Can you work these out from the model? Positions are in its coordinate system, mm. A direction names the side the tool comes from. Coordinates: 2 decimals unless noted, no trailing zeros. Loops run counter-clockwise (first coordinate to the right, second up) from the corner with the lowest first, then second, coordinate; pieces in that order, holes last.
Autodesk Fusion 360 part; units mm, degrees
box "BoxPrimitive1" add length 40 width 165 height 3.5 placed x (0, 1, 0) y (-1, 0, 0) z (0, 0, 1) at (165, 0, 0)
box "BoxPrimitive2" add length 40 width 2.5 height 23 placed x (0, 1, 0) y (-1, 0, 0) z (0, 0, 1) at (167.5, 0, 0)
hole "Hole1" at (167.5, 20.3218, 13.4545) direction (-1, 0, 0) diameter 6 depth 5 tip angle 180
Item 1: We'd pull the mould along Z, two halves only. Please class faces 1 (the face through (166.232, 17.792, 11.842)), 2 (the face through (84, 40, 1)), 3 (the face through (83, 20, 0)): +Z half, -Z half, draft (parallel to the pull), parting line (faces both ways), or undercut.
Results are:
face 1: undercut
face 2: draft
face 3: -Z half
Item 2: Suppose I cut it at B-B, the plane x = 42. Please give me the cut outline in (y, z).
Results are:
outline: (0, 0) - (40, 0) - (40, 3.5) - (0, 3.5) - close
Item 3: I need wall thicknesses on line 1 along Z through (x, y) = (43, 28); line 2 along X through (y, z) = (22, 17). Which ranges of each line are inside material? Lowest first, please.
Results are:
line 1: z = 0 to 3.5
line 2: x = 165 to 167.5
Item 4: Suppose I cut it at C-C, the plane z = 21.5. Please give me the cut outline in (x, y), plus the area to 3 significant figures.
Results are:
outline: (165, 0) - (167.5, 0) - (167.5, 40) - (165, 40) - close
area: 100 mm2
Item 5: On a 3-axis mill with a long thin cutter (end or side, diameter ignored), from which of +Z, -Z, +X, -X, +Y, -Y can I reach the whole of each face in a straight line? I mean faces 4 (the face through (0, 20, 2)), 5 (the face through (165, 20, 17)). Say none if no direction works.
Results are:
face 4: +Z, -Z, -X, +Y, -Y
face 5: +Z, -X, +Y, -Y
Item 6: I'm going to push flat-ended pins straight in: P1, Ø3, axis at x = 63, y = 31.5, coming from the +Z side; P2, Ø1, axis at y = 8, z = 20, coming from the -X side. Where does each tip first touch, or does it pass through?
Results are:
P1: stops at z = 3.5
P2: stops at x = 165
Item 7: Suppose I cut it at A-A, the plane y = 30.5. Please give me the cut outline in (x, z), plus the area to 3 significant figures.
Results are:
outline: (0, 0) - (167.5, 0) - (167.5, 23) - (165, 23) - (165, 3.5) - (0, 3.5) - close
area: 635 mm2
